Verification items for this drawing (mm, ordinates from the low corner). A direction names the side the tool comes from. Round coordinates to 2 decimals unless told otherwise and drop trailing zeros. Loops run counter-clockwise (first coordinate to the right, second up) from the corner with the lowest first, then second, coordinate; pieces in that order, holes last. Notation, with made-up numbers: M -17.75,32 L 41.25,32 A19 ccw 41.25,63 Z; hole C 13.25,40 d10. An arc over 180 degrees is marked long. Use one line per item in the form item = value. Start each with the question number.
1. Set-up check for the marked faces 5, 6 and 7: record each of +Z, -Z, +X, -X, +Y, -Y from which the full face is reachable in a straight line by a thin tool's end or side.
2. Go/stop test with flat-tipped pins: pin 1 (3 mm diameter, centred on y = 43, z = 45, fed in from -X); pin 2 (17 mm diameter, centred on x = 189.5, z = 17.5, fed in from -Y); pin 3 (4 mm diameter, centred on y = 66, z = 22, fed in from +X); pin 4 (17 mm diameter, centred on x = 17.5, z = 56.5, fed in from +Y). Record where each tip stops, or that it passes through.
3. Draft check along X on the marked faces 1, 2, 3 and 4. Enter one of: pulls with the +X half, pulls with the -X half, needs draft (parallel to the pull), parting line crosses it, or undercut.
4. Cross-section at C-C (x = 17.5). Record the boundary of the cut face in (y, z).
5. Cross-section at B-B (z = 17.5). Record the boundary of the cut face in (x, y).
6. Material ranges on line 1 (Z direction, x = 17, y = 34); line 2 (X direction, y = 39.5, z = 17.5); line 3 (X direction, y = 47, z = 39), recorded low to high.
7. Cross-section at A-A (y = 40). Record the boundary of the cut face in (x, z), then the cut area to 3 significant figures.
8. Cross-section at D-D (z = 6). Record the boundary of the cut face in (x, y), then the cut area to 3 significant figures.
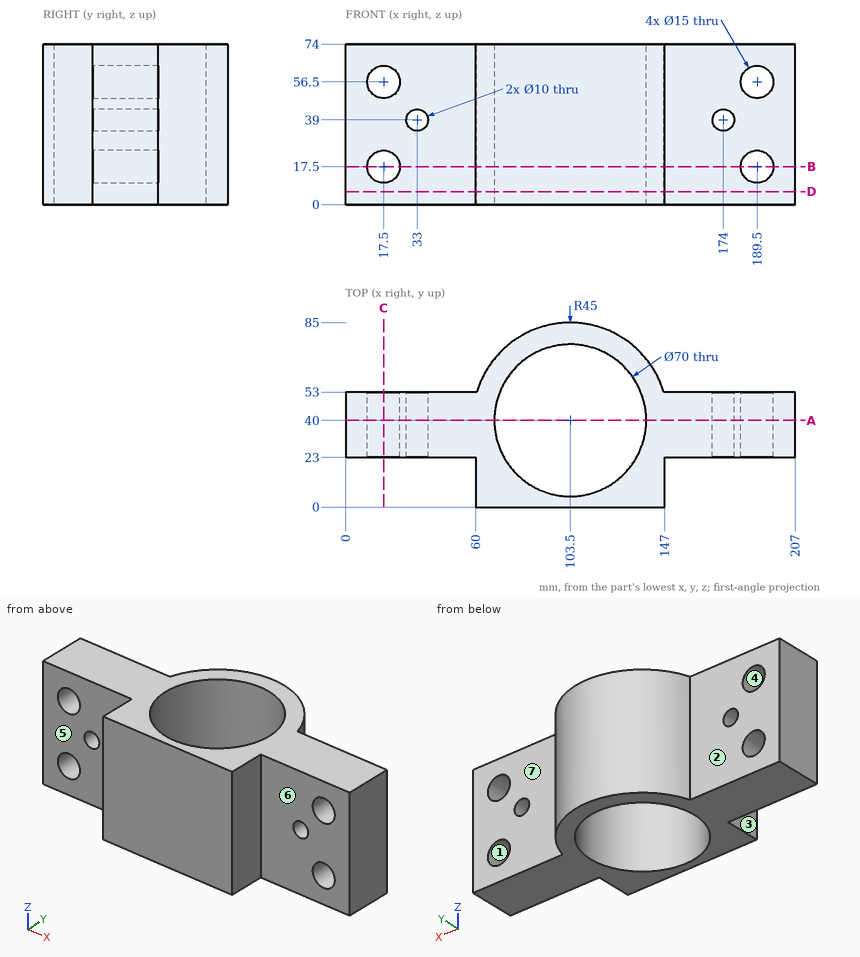
Reported:
q1.face_5 = +Z, -Z, -X, -Y
q1.face_6 = +Z, -Z, +X, -Y
q1.face_7 = +Z, -Z, +X, +Y
q2.pin_1 = 0
q2.pin_2 = 23
q2.pin_3 = 141.57
q2.pin_4 = 53
q3.face_1 = undercut
q3.face_2 = needs draft
q3.face_3 = pulls with the -X half
q3.face_4 = undercut
q4.outline = M 23,0 L 53,0 L 53,10 L 23,10 Z; M 23,25 L 53,25 L 53,49 L 23,49 Z; M 23,64 L 53,64 L 53,74 L 23,74 Z
q5.outline = M 0,23 L 10,23 L 10,53 L 0,53 Z; M 25,23 L 60,23 L 60,0 L 147,0 L 147,23 L 182,23 L 182,53 L 146.58,53 A45 ccw 60.42,53 L 25,53 Z; M 197,23 L 207,23 L 207,53 L 197,53 Z; hole C 103.5,40 d70
q6.line_1 = 0 to 10.02, 24.98 to 49.02, 63.98 to 74
q6.line_2 = 0 to 10, 25 to 68.5, 138.5 to 182, 197 to 207
q6.line_3 = 0 to 28, 38 to 69.21, 137.79 to 169, 179 to 207
q7.outline = M 0,0 L 68.5,0 L 68.5,74 L 0,74 Z; M 138.5,0 L 207,0 L 207,74 L 138.5,74 Z; hole C 17.5,17.5 d15; hole C 17.5,56.5 d15; hole C 33,39 d10; hole C 174,39 d10; hole C 189.5,17.5 d15; hole C 189.5,56.5 d15
q7.area = 9,270 mm²
q8.outline = M 0,23 L 60,23 L 60,0 L 147,0 L 147,23 L 207,23 L 207,53 L 146.58,53 A45 ccw 60.42,53 L 0,53 Z; hole C 103.5,40 d70
q8.area = 6,390 mm²
